from build123d import *

# Parameters (mm, degrees)
SKETCH1_W           = 55
SKETCH1_H           = 8
BOSS_EXTRUDE1_DEPTH = 16
SKETCH2_R           = 2.5
CUT_EXTRUDE1_DEPTH  = 16
SKETCH3_W           = 55
SKETCH3_H           = 16
BOSS_EXTRUDE2_DEPTH = 4
SKETCH4_W           = 55
SKETCH4_H           = 16
BOSS_EXTRUDE3_DEPTH = 4


with BuildPart() as part:
    # Sketch1 → Boss-Extrude1 (new body)
    with BuildSketch(Plane(origin=(0, 0, 0), x_dir=(1, 0, 0), z_dir=(0, 1, 0))):
        with Locations((27.5, 4)):
            Rectangle(SKETCH1_W, SKETCH1_H)
    extrude(amount=BOSS_EXTRUDE1_DEPTH)

    # Sketch2 → Cut-Extrude1 (cut)
    with BuildSketch(Plane(origin=(0, 16, 0), x_dir=(1, 0, 0), z_dir=(0, 1, 0))):
        with Locations(Location((6.5, 4, 0), (0, 0, 270))):
            Circle(SKETCH2_R)
        with Locations(Location((48.5, 4, 0), (0, 0, 270))):
            Circle(SKETCH2_R)
    extrude(amount=-CUT_EXTRUDE1_DEPTH, mode=Mode.SUBTRACT)

    # Sketch3 → Boss-Extrude2 (add)
    with BuildSketch(Plane.XY):
        with Locations((27.5, 8)):
            Rectangle(SKETCH3_W, SKETCH3_H)
    extrude(amount=BOSS_EXTRUDE2_DEPTH)

    # Sketch4 → Boss-Extrude3 (add)
    with BuildSketch(Plane(origin=(0, 0, -8), x_dir=(-1, 0, 0), z_dir=(0, 0, -1))):
        with Locations((-27.5, 8)):
            Rectangle(SKETCH4_W, SKETCH4_H)
    extrude(amount=BOSS_EXTRUDE3_DEPTH)


solid = part.part
The listing builds one solid part. Answer for the finished solid, in the listing's coordinates (mm). Round coordinates to 2 decimals unless told otherwise and drop trailing zeros. Write each loop counter-clockwise with the first axis right and the second up, starting at its lowest first coordinate (ties: lowest second). Pieces come first, ordered by that corner, then holes. Notation, with made-up numbers: (78.5, 87) - (82.5, 87) arc R28 cw to (82.5, 122) - close; hole circle Ø6 at (85, -13). An arc over 180 degrees is marked (long way). Use one line per item in the form item = value. Start each with the question number.
Item 1: A flat-ended cylindrical pin translates along its axis: pin 1 Ø4 at (x, z) = (48.5, -4) entering from +Y. Find the tip coordinate at first contact, or state that the pin passes through.
Item 2: Determine the mould class of faces 1 (the cylindrical face through (7.251, 8.112, -1.615)), 2 (the flat face through (28, 0, -4)), 3 (the flat face through (0, 8, -4)) for opening direction X: +X half, -X half, draft (parallel to the pull), parting line (faces both ways), or undercut.
Item 3: A cutting plane is placed at A-A (x = 6.5). Write down the section's boundary in (y, z).
Item 4: A cutting plane is placed at C-C (z = -4). Write down the section's boundary in (x, y), plus the area to 3 significant figures.
Item 5: A cutting plane is placed at B-B (y = 15). Write down the section's boundary in (x, z), plus the area to 3 significant figures.
Item 6: Find the intervals of material crossed by line 1 (X direction, y = 10.25, z = -4); line 2 (X direction, y = 11.25, z = -2.5), in increasing order. Write a range as [from, to].
Item 7: A cutting plane is placed at D-D (x = 50). Write down the section's boundary in (y, z), plus the area to 3 significant figures.
The answers:
q1.pin_1 = through
q2.face_1 = undercut
q2.face_2 = draft
q2.face_3 = -X half
q3.outline = (0, -12) - (16, -12) - (16, -6.5) - (0, -6.5) - close; (0, -1.5) - (16, -1.5) - (16, 4) - (0, 4) - close
q4.outline = (0, 0) - (4, 0) - (4, 16) - (0, 16) - close; (9, 0) - (46, 0) - (46, 16) - (9, 16) - close; (51, 0) - (55, 0) - (55, 16) - (51, 16) - close
q4.area = 720 mm^2
q5.outline = (0, -12) - (55, -12) - (55, 4) - (0, 4) - close; hole circle Ø5 at (6.5, -4); hole circle Ø5 at (48.5, -4)
q5.area = 841 mm^2
q6.line_1 = [0, 4], [9, 46], [51, 55]
q6.line_2 = [0, 4.5], [8.5, 46.5], [50.5, 55]
q7.outline = (0, -12) - (16, -12) - (16, -6) - (0, -6) - close; (0, -2) - (16, -2) - (16, 4) - (0, 4) - close
q7.area = 192 mm^2
